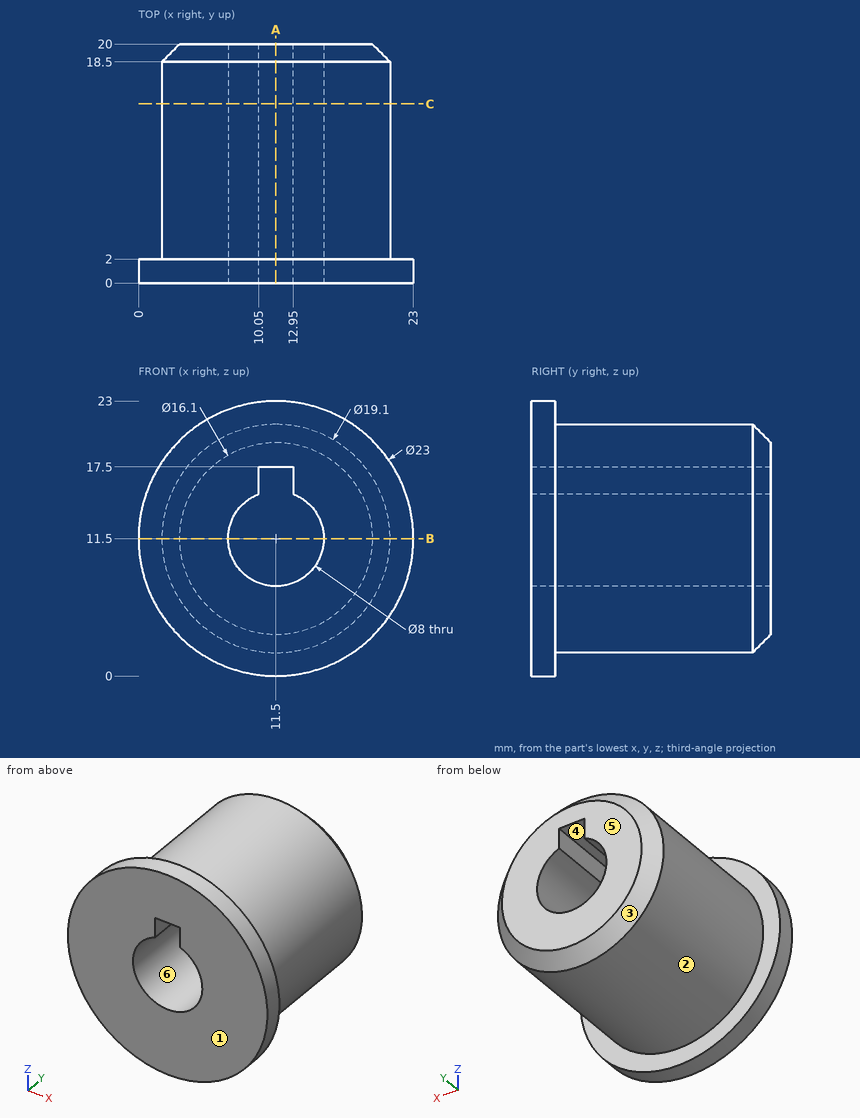
The drawing under review shows one solid part. Ordinate dimensions are in mm from its lowest x, y, z. A direction names the side the tool comes from. Round coordinates to 2 decimals unless told otherwise and drop trailing zeros. Loops run counter-clockwise (first coordinate to the right, second up) from the corner with the lowest first, then second, coordinate; pieces in that order, holes last. Notation, with made-up numbers: (-18.75, 22) -> (9.25, 22) arc R23 cw to (9.25, 31) -> close; hole circle Ø8 at (18.5, -4). An arc over 180 degrees is marked (long way). One line per question, with ' | ' between items. Start each with the question number.
Item 1: Wall thickness on line 1 along X through (y, z) = (8.75, 11.5); line 2 along Z through (x, y) = (11.5, 7.25); line 3 along Y through (x, z) = (6.5, 2.75): over which ranges is each line inside the solid? List them lowest first. Write a range as [from, to].
Item 2: Machinability: for the marked faces 1 and 2, which of the approach directions +Z, -Z, +X, -X, +Y, -Y give a long, thin tool a straight path to every point of the face, cutting with its end or side? Answer none if there is none.
Item 3: For pin 1 (10 mm diameter, centred on x = 8.5, z = 13, fed in from -Y); pin 2 (6 mm diameter, centred on y = 5.5, z = 8, fed in from +X); pin 3 (1.5 mm diameter, centred on x = 15, y = 10.5, fed in from +Z); pin 4 (2 mm diameter, centred on x = 5, y = 11, fed in from -Z), all flat-tipped, find the tip position at first contact; note any pin that passes through.
Item 4: Add section C-C, the plane y = 15. Write out the cut boundary in (x, z).
Item 5: Draft analysis for pull direction X (two halves, no side actions). For the marked faces 3, 4, 5 and 6, state which applies: +X half, -X half, draft (parallel to the pull), parting line (faces both ways), or undercut.
Item 6: Add section B-B, the plane z = 11.5. Write out the cut boundary in (x, y), then the cut area to 3 significant figures.
Item 7: Add section A-A, the plane x = 11.5. Write out the cut boundary in (y, z), then the cut area to 3 significant figures.
Return value:
1) line 1: x = [1.95, 7.5], [15.5, 21.05] | line 2: z = [1.95, 7.5], [17.5, 21.05] | line 3: y = [0, 2]
2) face 1: +Z, -Z, +X, -X, -Y | face 2: +Y
3) pin 1: stops at y = 0 | pin 2: stops at x = 21.04 | pin 3: stops at z = 20.65 | pin 4: stops at z = 3.69
4) outline: circle Ø19.1 at (11.5, 11.5); hole (10.05, 15.23) arc R4 ccw (long way) to (12.95, 15.23) -> (12.95, 17.5) -> (10.05, 17.5) -> close
5) face 3: parting line | face 4: undercut | face 5: draft | face 6: undercut
6) outline: (0, 0) -> (7.5, 0) -> (7.5, 20) -> (3.45, 20) -> (1.95, 18.5) -> (1.95, 2) -> (0, 2) -> close; (15.5, 0) -> (23, 0) -> (23, 2) -> (21.05, 2) -> (21.05, 18.5) -> (19.55, 20) -> (15.5, 20) -> close | area: 228 mm2
7) outline: (0, 0) -> (2, 0) -> (2, 1.95) -> (18.5, 1.95) -> (20, 3.45) -> (20, 7.5) -> (0, 7.5) -> close; (0, 17.5) -> (20, 17.5) -> (20, 19.55) -> (18.5, 21.05) -> (2, 21.05) -> (2, 23) -> (0, 23) -> close | area: 188 mm2
